from build123d import *

# Parameters (mm, degrees)
SKETCH1_R                  = 34.384
SKETCH1_R_2                = 24.384
BOSS_EXTRUDE1_DEPTH        = 35
BOSS_EXTRUDE2_START        = -10
SKETCH1_3_R                = 34.384
BOSS_EXTRUDE2_DEPTH        = 10
SKETCH3_R                  = 12.5
BOSS_EXTRUDE3_DEPTH        = 10
FILLET1_R                  = 5
F_12_0MM_DOWEL_HOLE1_D     = 11
F_12_0MM_DOWEL_HOLE1_DEPTH = 10
F_8_0MM_DOWEL_HOLE2_D      = 9
CHAMFER1_SIZE              = 2
CHAMFER2_SIZE              = 0.5
CHAMFER4_SIZE              = 0.5
FILLET2_R                  = 5


with BuildPart() as part:
    # Sketch1 → Boss-Extrude1 (new body)
    with BuildSketch(Plane(origin=(0, 0, 0), x_dir=(1, 0, 0), z_dir=(0, 1, 0))):
        with Locations(Location((0, 0, 0), (0, 0, 270))):
            Circle(SKETCH1_R)
        with Locations(Location((0, 0, 0), (0, 0, 270))):
            Circle(SKETCH1_R_2, mode=Mode.SUBTRACT)
    extrude(amount=BOSS_EXTRUDE1_DEPTH)

    # Sketch1<3> → Boss-Extrude2 (add)
    with BuildSketch(Plane(origin=(0, 0, 0), x_dir=(1, 0, 0), z_dir=(0, 1, 0)).offset(BOSS_EXTRUDE2_START)):
        with Locations(Location((0, 0, 0), (0, 0, 270))):
            Circle(SKETCH1_3_R)
    extrude(amount=BOSS_EXTRUDE2_DEPTH)

    # Sketch3 → Boss-Extrude3 (add)
    with BuildSketch(Plane(origin=(0, 0, 0), x_dir=(1, 0, 0), z_dir=(0, 1, 0))):
        with Locations(Location((0, 0, 0), (0, 0, 270))):
            Circle(SKETCH3_R)
    extrude(amount=BOSS_EXTRUDE3_DEPTH)

    # Fillet1
    fillet1_edges = [part.edges().sort_by_distance(p)[0] for p in [
        (0, 0, -12.5),
        (0, 10, -12.5),
    ]]
    fillet(fillet1_edges, radius=FILLET1_R - 0.0001)  # a hair under: the kernel refuses the full size

    # Ø12.0mm Dowel Hole1
    with Locations(Plane(origin=(0, -10, 0), x_dir=(-1, 0, 0), z_dir=(0, -1, 0))):
        with Locations((0, 0)):
            Hole(F_12_0MM_DOWEL_HOLE1_D / 2, depth=F_12_0MM_DOWEL_HOLE1_DEPTH)

    # Ø8.0mm Dowel Hole2 (through all)
    with Locations(Plane(origin=(0, 0, 0), x_dir=(-1, 0, 0), z_dir=(0, -1, 0))):
        with Locations((0, 0)):
            Hole(F_8_0MM_DOWEL_HOLE2_D / 2)

    # Chamfer1
    chamfer1_edges = [part.edges().sort_by_distance(p)[0] for p in [
        (0, 35, -24.384),
    ]]
    chamfer(chamfer1_edges, length=CHAMFER1_SIZE)

    # Chamfer2
    chamfer2_edges = [part.edges().sort_by_distance(p)[0] for p in [
        (-5.5, -10, 0),
    ]]
    chamfer(chamfer2_edges, length=CHAMFER2_SIZE)

    # Chamfer4
    chamfer4_edges = [part.edges().sort_by_distance(p)[0] for p in [
        (-5.5, 0, 0),
        (-4.5, 0, 0),
    ]]
    chamfer(chamfer4_edges, length=CHAMFER4_SIZE - 0.0001)  # a hair under: the kernel refuses the full size

    # Fillet2
    fillet2_edges = [part.edges().sort_by_distance(p)[0] for p in [
        (0, 35, -26.384),
        (0, 35, -34.384),
    ]]
    fillet(fillet2_edges, radius=FILLET2_R)


solid = part.part
Source: CAD feature listing. Evaluate the final solid. Frame: model axes, mm. A direction names the side the tool comes from. Give positions to 0.01 mm unless a question says otherwise; leave off trailing zeros. Order: outer loops, then holes, each group sorted by start corner. A loop starts at its lowest first (then second) coordinate and runs counter-clockwise, first axis right, second up. Notation, with made-up numbers: (1, 44.25) -> (30, 44.25) arc R25 cw to (30, 58.25) -> close; hole circle Ø7 at (-8.5, 87.5). An arc over 180 degrees is marked (long way). Write item = value, one per line.
Q1. Cut plane B-B, the plane y = -6.5. Output: boundary loops of the cut face in (x, z), and give its area (3 significant figures).
Data:
outline = circle Ø68.77 at (0, 0); hole circle Ø11 at (0, 0)
area = 3,620 mm^2
Q2. Set-up query: faces 1 (the face through (-5, 10, 0)), 2 (the face through (-1.19, -4.94, 5.37)), 3 (the face through (-0.59, 5.32, -4.46)). Return all of +Z, -Z, +X, -X, +Y, -Y with unobstructed straight access to the full face (end or side cutting, diameter ignored); none if empty.
Data:
face_1 = +Y
face_2 = -Y
face_3 = +Y, -Y
Q3. Pull-direction query (X, two-part tool) for faces 4 (the face through (17, 0, -6)), 5 (the face through (0, -10, 7)), 6 (the face through (10.328, 9.72, 32.796)); classes: released by +X, released by -X, zero draft, split by the parting line, or undercut.
Data:
face_4 = undercut
face_5 = zero draft
face_6 = split by the parting line
Q4. Material intervals for line 1 (X direction, y = 9, z = 0); line 2 (X direction, y = -7.5, z = 0); line 3 (Z direction, x = -17, y = 20), sorted ascending. Write a range as from..to.
Data:
line_1 = -34.38..-24.38, -10.5..-4.5, 4.5..10.5, 24.38..34.38
line_2 = -34.38..-5.5, 5.5..34.38
line_3 = -29.89..-17.48, 17.48..29.89
Q5. Pin query (flat end, axial travel): pin 1 (12 mm diameter, centred on x = 7, z = -18, fed in from +Y); pin 2 (1.5 mm diameter, centred on x = -9, y = 0.5, fed in from -Z); pin 3 (5 mm diameter, centred on y = 23.5, z = -4.5, fed in from +X). Return the tip coordinate at first contact, or that it passes through.
Data:
pin_1 = 33.89
pin_2 = -33.38
pin_3 = 34.33
Q6. Cut plane A-A, the plane y = 11. Output: boundary loops of the cut face in (x, z).
Data:
outline = circle Ø68.77 at (0, 0); hole circle Ø48.77 at (0, 0)
